Work out the finished part from the listing and answer in its coordinate system (mm). Face numbers are marked on the shaded views. A direction names the side the tool comes from. Coordinates: 2 decimals unless noted, no trailing zeros. Loops run counter-clockwise (first coordinate to the right, second up) from the corner with the lowest first, then second, coordinate; pieces in that order, holes last. Notation, with made-up numbers: M -7,20 L 47,20 A33 cw 47,58 Z; hole C 27.25,-10 d4. An arc over 180 degrees is marked long. Write each question's results on one line, items separated by ' | '.
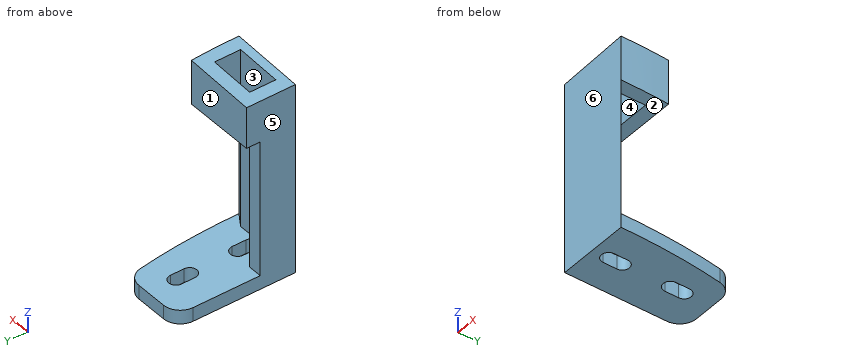
```python
from build123d import *

# Parameters (mm, degrees)
BOSS_EXTRUDE1_DEPTH = 3.175
BOSS_EXTRUDE2_DEPTH = 41.15
SKETCH3_W           = 10.5
SKETCH3_H           = 6
BOSS_EXTRUDE3_DEPTH = 10.16
CUT_EXTRUDE1_DEPTH  = 39.555801056


with BuildPart() as part:
    # Sketch1 → Boss-Extrude1 (new body)
    with BuildSketch(Plane.XY):
        with BuildLine():
            Line((71.045544716, 27.335394647), (63.656604316, 27.335394647))
            ThreePointArc((63.656604316, 27.335394647), (60.962527479, 26.219471483), (59.846604316, 23.525394647))
            Line((59.846604316, 23.525394647), (59.846604316, -23.525394647))
            ThreePointArc((59.846604316, -23.525394647), (60.962527479, -26.219471483), (63.656604316, -27.335394647))
            Line((63.656604316, -27.335394647), (71.045544716, -27.335394647))
            ThreePointArc((71.045544716, -27.335394647), (73.499934786, -26.439510188), (74.800072929, -24.173173852))
            add(Edge.make_bspline(
                [(76.701202739, 0), (76.701202739, -8.04022214), (76.161781205, -16.280712803), (74.800072929, -24.173173852)],
                knots=[0, 0, 0, 0, 0.259951787, 0.259951787, 0.259951787, 0.259951787], degree=3))
            add(Edge.make_bspline(
                [(74.800072929, 24.173173852), (76.161781205, 16.280712803), (76.701202739, 8.04022214), (76.701202739, 0)],
                knots=[0.740048213, 0.740048213, 0.740048213, 0.740048213, 1, 1, 1, 1], degree=3))
            ThreePointArc((74.800072929, 24.173173852), (73.499934786, 26.439510188), (71.045544716, 27.335394647))
        make_face()
        with BuildLine():
            Line((66.641953527, -20.985394647), (66.641953527, -17.810394647))
            ThreePointArc((66.641953527, -17.810394647), (68.273903527, -16.178444647), (69.905853527, -17.810394647))
            Line((69.905853527, -17.810394647), (69.905853527, -20.985394647))
            ThreePointArc((69.905853527, -20.985394647), (68.273903527, -22.617344647), (66.641953527, -20.985394647))
        make_face(mode=Mode.SUBTRACT)
        with BuildLine():
            Line((66.497091774, -6.896821773), (66.497091774, -3.721821773))
            ThreePointArc((66.497091774, -3.721821773), (68.129041774, -2.089871773), (69.760991774, -3.721821773))
            Line((69.760991774, -3.721821773), (69.760991774, -6.896821773))
            ThreePointArc((69.760991774, -6.896821773), (68.129041774, -8.528771773), (66.497091774, -6.896821773))
        make_face(mode=Mode.SUBTRACT)
        with BuildLine():
            Line((66.641953527, 20.985394647), (66.641953527, 17.810394647))
            ThreePointArc((66.641953527, 17.810394647), (68.273903527, 16.178444647), (69.905853527, 17.810394647))
            Line((69.905853527, 17.810394647), (69.905853527, 20.985394647))
            ThreePointArc((69.905853527, 20.985394647), (68.273903527, 22.617344647), (66.641953527, 20.985394647))
        make_face(mode=Mode.SUBTRACT)
        with BuildLine():
            Line((66.497091774, 6.896821773), (66.497091774, 3.721821773))
            ThreePointArc((66.497091774, 3.721821773), (68.129041774, 2.089871773), (69.760991774, 3.721821773))
            Line((69.760991774, 3.721821773), (69.760991774, 6.896821773))
            ThreePointArc((69.760991774, 6.896821773), (68.129041774, 8.528771773), (66.497091774, 6.896821773))
        make_face(mode=Mode.SUBTRACT)
    extrude(amount=BOSS_EXTRUDE1_DEPTH)

    # Sketch2 → Boss-Extrude2 (add)
    with BuildSketch(Plane.XY.offset(3.175)):
        Polygon((76.701202739, 0), (73.487010624, 2.08), (62.987010624, 2.08), (62.987010624, 8.08), (59.846604316, 8.08), (59.846604316, -8.08), (62.987010624, -8.08), (62.987010624, -2.08), (73.487010624, -2.08), align=None)
    extrude(amount=BOSS_EXTRUDE2_DEPTH)

    # Sketch3 → Boss-Extrude3 (add)
    with BuildSketch(Plane.XY.offset(44.325)):
        with BuildLine():
            Line((59.846604316, 8.08), (59.846604316, 11.220406309))
            Line((59.846604316, 11.220406309), (76.327728698, 11.220406308))
            add(Edge.make_bspline(
                [(76.701202739, 0), (76.701202739, 3.71540513), (76.586015455, 7.473575307), (76.327728698, 11.220406308)],
                knots=[0, 0, 0, 0, 0.120124318, 0.120124318, 0.120124318, 0.120124318], degree=3))
            add(Edge.make_bspline(
                [(76.701202739, 0), (76.701202739, -3.71540513), (76.586015455, -7.473575307), (76.327728698, -11.220406308)],
                knots=[0, 0, 0, 0, 0.120124318, 0.120124318, 0.120124318, 0.120124318], degree=3))
            Line((76.327728698, -11.220406308), (59.846604316, -11.220406309))
            Line((59.846604316, -11.220406309), (59.846604316, -8.08))
            Line((59.846604316, -8.08), (59.846604316, 8.08))
        make_face()
        with Locations((68.237010624, 5.08)):
            Rectangle(SKETCH3_W, SKETCH3_H, mode=Mode.SUBTRACT)
        with Locations((68.237010624, -5.08)):
            Rectangle(SKETCH3_W, SKETCH3_H, mode=Mode.SUBTRACT)
    extrude(amount=-BOSS_EXTRUDE3_DEPTH)

    # Sketch4 → Cut-Extrude1 (cut, through all)
    with BuildSketch(Plane(origin=(0, 11.220406309, 0), x_dir=(1, 0, 0), z_dir=(0, 1, 0))):
        Polygon((76.701202739, -44.325), (59.846604316, -43.589112341), (59.846604316, -44.325), align=None)
    extrude(amount=-CUT_EXTRUDE1_DEPTH, mode=Mode.SUBTRACT)


with BuildPart() as body_2:
    # Split1: the piece on the far side of the plane
    add(part.part)
    split(bisect_by=Plane(origin=(0, 0, 0), x_dir=(1, 0, 0), z_dir=(0, 1, 0)), keep=Keep.BOTTOM)


with BuildPart() as part_1:
    add(part.part)

    # Split1
    split(bisect_by=Plane(origin=(0, 0, 0), x_dir=(1, 0, 0), z_dir=(0, 1, 0)), keep=Keep.TOP)


solid = part_1.part
```
1) Find section D-D, the plane y = 25.25. Give the vertices of the cut face in (x, z) (3 decimals).
Check result:
outline: M 60.259,0 L 74.443,0 L 74.443,3.175 L 60.259,3.175 Z
2) For a pull along X with two mould halves and no side action, classify the marked faces 4, 5 and 6 as released by +X, released by -X, zero draft, split by the parting line, or undercut.
Check result:
face 4: undercut | face 5: released by -X | face 6: zero draft
3) Find section B-B, the plane z = 28.5. Give the vertices of the cut face in (x, y), and give its area (3 significant figures).
Check result:
outline: M 59.85,0 L 76.7,0 L 73.49,2.08 L 62.99,2.08 L 62.99,8.08 L 59.85,8.08 Z | area: 50.6 mm^2
4) Which of the six approach directions +Z, -Z, +X, -X, +Y, -Y give full straight-line access (tool end or side, diameter ignored) to the marked faces 1, 2 and 3?
Check result:
face 1: +Z, +X, -X, +Y | face 2: +X, +Y | face 3: +Z
5) Find section A-A, the plane x = 65.25. Give the vertices of the cut face in (y, z) (3 decimals), and give its area (3 significant figures).
Check result:
outline: M 0,0 L 27.335,0 L 27.335,3.175 L 2.08,3.175 L 2.08,43.825 L 0,43.825 Z; M 8.08,34.165 L 11.22,34.165 L 11.22,43.825 L 8.08,43.825 Z | area: 202 mm^2
6) Given pin 1 Ø10 at (x, y) = (67, 14) entering from -Z; pin 2 Ø5 at (x, z) = (67, 39) entering from +Y; pin 3 Ø8 at (y, z) = (13.5, 33.5) entering from +X; pin 4 Ø4 at (x, z) = (64.5, 11) entering from +Y, each flat-ended and moving along its own axis, determine where each tip first touches the part or whether it passes through.
Check result:
pin 1: z = 0 | pin 2: y = 11.22 | pin 3: x = 76.43 | pin 4: y = 8.08
7) Find section C-C, the plane x = 70.5. Give the vertices of the cut face in (y, z) (3 decimals).
Check result:
outline: M 0,0 L 27.335,0 L 27.335,3.175 L 2.08,3.175 L 2.08,44.054 L 0,44.054 Z; M 8.08,34.165 L 11.22,34.165 L 11.22,44.054 L 8.08,44.054 Z
8) Straight lines are drawn through the part: probe 1 along Y at (x, z) = (65, 36); probe 2 along Y at (x, z) = (69.5, 3); probe 3 along Z at (x, y) = (63, 26) (3 decimals). For each, find the intervals that lie inside material, in ascending order. Write a range as [from, to].
Check result:
probe 1: [0, 2.08], [8.08, 11.22] | probe 2: [0, 2.84], [7.78, 16.73], [22.06, 27.34] | probe 3: [0, 3.175]
